Check sheet for the drawn part. Datum: minimum x, y, z corner. Units: mm. Coordinates: 2 decimals unless noted, no trailing zeros. Write each loop counter-clockwise with the first axis right and the second up, starting at its lowest first coordinate (ties: lowest second). Pieces come first, ordered by that corner, then holes. Notation, with made-up numbers: (84, 74) -> (128, 74) arc R19 cw to (128, 109) -> close; hole circle Ø1 at (-13.75, -28.75). An arc over 180 degrees is marked (long way). Answer in a Markdown table with one row per item.
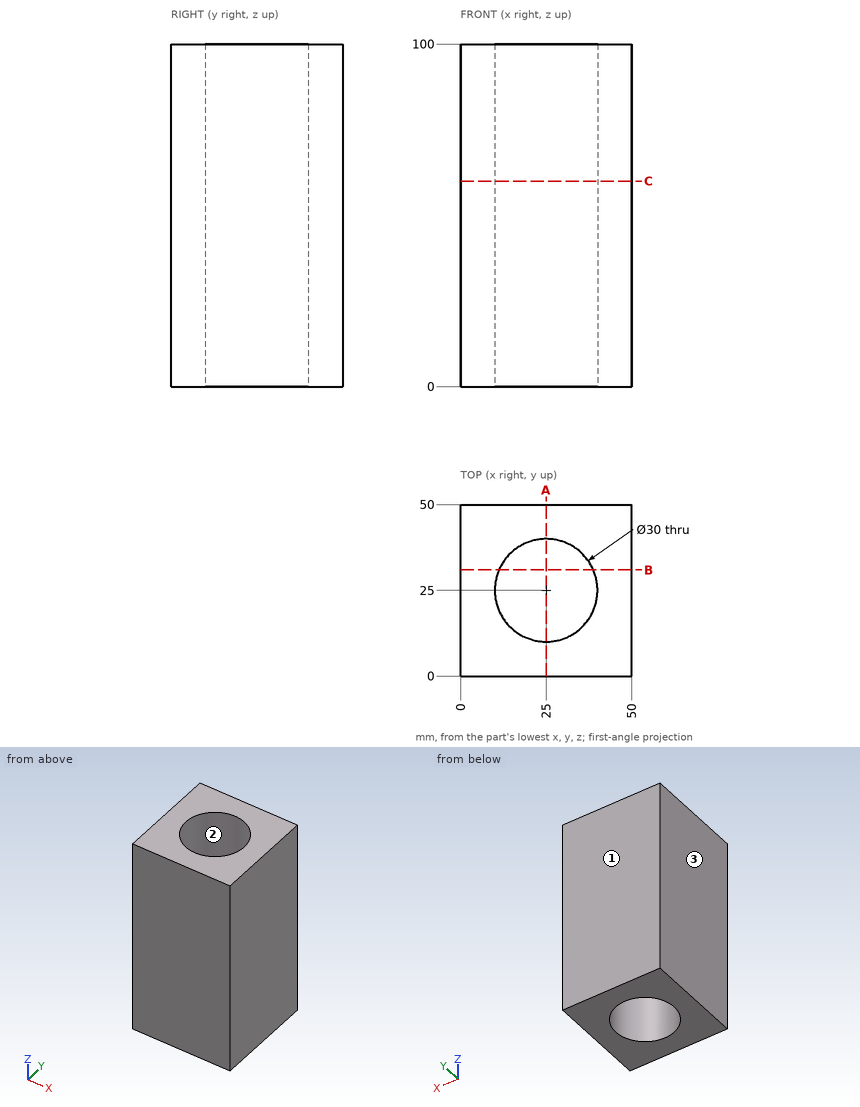
1. Release check for a two-part mould opening along X. For the marked faces 1, 2 and 3 record: released by +X, released by -X, zero draft, split by the parting line, or undercut.
Findings below:
| item | result |
|---|---|
| face 1 | zero draft |
| face 2 | undercut |
| face 3 | released by -X |
2. Sectioned sample at A-A, the plane x = 25. Record the cut outline in (y, z).
Findings below:
| item | result |
|---|---|
| outline | (0, 0) -> (10, 0) -> (10, 100) -> (0, 100) -> close; (40, 0) -> (50, 0) -> (50, 100) -> (40, 100) -> close |
3. Material ranges on probe 1 along Y at (x, z) = (25, 31); probe 2 along X at (y, z) = (32.5, 29); probe 3 along X at (y, z) = (12, 44), recorded low to high. Write a range as from..to.
Findings below:
| item | result |
|---|---|
| probe 1 | y = 0..10, 40..50 |
| probe 2 | x = 0..12.01, 37.99..50 |
| probe 3 | x = 0..17.52, 32.48..50 |
4. Sectioned sample at B-B, the plane y = 31. Record the cut outline in (x, z), and give its area (3 significant figures).
Findings below:
| item | result |
|---|---|
| outline | (0, 0) -> (11.25, 0) -> (11.25, 100) -> (0, 100) -> close; (38.75, 0) -> (50, 0) -> (50, 100) -> (38.75, 100) -> close |
| area | 2,250 mm² |
5. Sectioned sample at C-C, the plane z = 60. Record the cut outline in (x, y).
Findings below:
| item | result |
|---|---|
| outline | (0, 0) -> (50, 0) -> (50, 50) -> (0, 50) -> close; hole circle Ø30 at (25, 25) |
